For this review, take the finished solid that the model builds, in its own axes (mm). Face numbers are marked on the shaded views. A direction names the side the tool comes from. Give positions to 0.01 mm unless a question says otherwise; leave off trailing zeros. Write each loop counter-clockwise with the first axis right and the second up, starting at its lowest first coordinate (ties: lowest second). Pieces come first, ordered by that corner, then holes. Notation, with made-up numbers: (-30, 10) -> (26, 10) arc R8 cw to (26, 15) -> close; hole circle Ø10 at (-26.75, -16). An arc over 180 degrees is marked (long way). Return JSON: item names as keys, results as strings.
Autodesk Inventor part; units mm, degrees
ref_plane "Work Plane1" through (1.525, 0, 0) normal (0, 0, 1) x (1, 0, 0)
ref_plane "YZ Plane" through (0, 0, 0) normal (1, 0, 0) x (0, 1, 0)
ref_plane "XZ Plane" through (0, 0, 0) normal (0, 1, 0) x (-1, 0, 0)
sketch "Sketch1" plane through (0, 0, 0) normal (0, 0, 1) x (1, 0, 0)
  line L0 (0, 15) -> (0, 10)
  line L1 (7.5, 10) -> (80, 10)
  line L2 (80, 10) -> (80, 0)
  line L3 (80, 0) -> (-0.8001, 0)
  line L4 (-16.9601, 0) -> (96.16, 0)
  line L5 (-0.8001, 0) -> (-0.8001, 15)
  line L6 (-0.8001, 15) -> (0, 15)
  line L7 (7.5, 10) -> (5.9663, 10)
  line L8 (5.9663, 10) -> (0, 10)
  line L9 (0, -3) -> (0, 18)
  dimension "d0" = 80
  dimension "d1" = 72.5
  dimension "d2" = 20
  dimension "d9" = 0.8001
  dimension "d10" = 30
  dimension "d13" = 1.5337
  dimension "d14" = 20
revolve "Body" add sketch "Sketch1" angle 360 about axis through (80, 0, 0) along (-1, 0, 0)
sketch "Sketch2" plane through (-0.8001, 0, 0) normal (-1, 0, 0) x (0, 0, 1)
  line L0 (0, 17.3205) -> (15, 8.6603)
  line L1 (15, 8.6603) -> (15, -8.6603)
  line L2 (15, -8.6603) -> (0, -17.3205)
  line L3 (0, -17.3205) -> (-15, -8.6603)
  line L4 (-15, -8.6603) -> (-15, 8.6603)
  line L5 (-15, 8.6603) -> (0, 17.3205)
  point P0 (0, 0)
  point P1 (0, 0)
  dimension "d11" = 30
extrude "Head" add sketch "Sketch2" along normal blind 11.7
sketch "Sketch4" plane through (0, 0, 0) normal (0, 0, 1) x (1, 0, 0)
  line L0 (-12.5001, 15) -> (-12.5001, 17.3205)
  line L1 (-12.5001, 17.3205) -> (-11.1604, 17.3205)
  line L2 (-11.1604, 17.3205) -> (-12.5001, 15)
  line L3 (-14.8401, 0) -> (1.5399, 0)
  line L4 (-0.8001, 17.3205) -> (-12.5001, 17.3205)
  line L5 (-12.5001, 8.6603) -> (-12.5001, 17.3205)
  dimension "d5" = 30
  dimension "d19" = 30
revolve "Chamfer1" cut sketch "Sketch4" angle 360 about axis through (-10, 0, 0) along (1, 0, 0)
thread "Thread"
chamfer "Chamfer2" distance 1.5336 distance2 1.5337 1 edges at (80, -10, 0) measured on face at (80, -2.8768, 3.7595)
ref_plane "Work Plane1" through (1.525, 0, 0) normal (0, 0, 1) x (1, 0, 0)
sketch "Sketch7" plane through (-12.5001, 0, 0) normal (-1, 0, 0) x (0, 0, 1)
  circle A0 centre (0, 0) radius 4.5
  dimension "d59" = 9
extrude "Extrusion5" cut sketch "Sketch7" against normal blind 45
equation "\"d11\" = SW"
equation "\"d3\" = KOH - SD"
equation "\"d15\" = GEL"
equation "\"d6\" = -0.5 * SPD + 0.5 * GD"
equation "\"d0\" = NLG"
equation "\"d1\" = GEL"
equation "\"d2\" = GD"
equation "\"d10\" = SD2"
equation "\"d14\" = BDM"
equation "\"d5\" = ANG1"
equation "\"d19\" = SW0"
equation "\"NLG\" = 80"
equation "\"GD\" = NND"
equation "\"BDM\" = NND"
equation "\"KOH\" = 12.5"
equation "\"GEL\" = 72.5"
equation "\"SW\" = 30"
equation "\"SW0\" = SW"
equation "\"SPD\" = NND - 1.2269 * PTC"
equation "\"SD2\" = SW"
equation "\"SD\" = 0.8"
equation "\"ANG1\" = 30deg"
equation "\"GAL\" = 0.61345 * PTC"
equation "\"GUL\" = 0.61345 * PTC"
equation "\"RR\" = 0.8"
equation "\"WFT\" = SD"
equation "\"GD1\" = THREADDIA - 1.2269 * PTC"
equation "\"TOA\" = 30deg"
equation "\"FAWI\" = 45deg"
equation "\"PTC\" = 2.5"
equation "\"E0\" = 1.155 * SW"
properties part number "AS 1110 - M20 x 80" material "Steel, Mild"
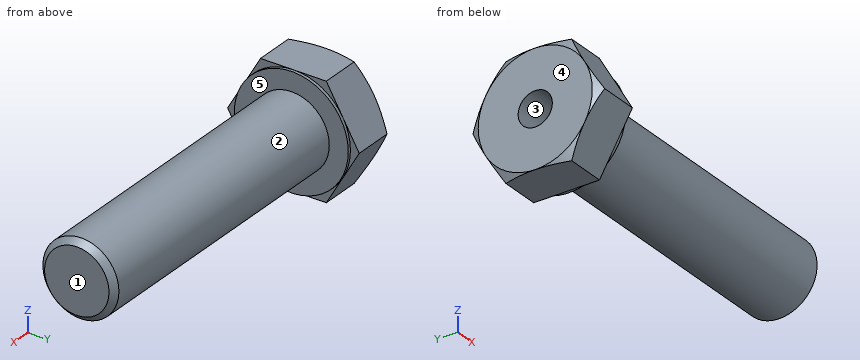
1. To check wall thickness, follow probe 1 along Y at (x, z) = (11, 0); probe 2 along X at (y, z) = (1.5, 12); probe 3 along X at (y, z) = (3, -2.5). State the ranges of each line that lie inside material, in increasing order.
Results found:
{"probe 1": "y = -10 to -4.5, 4.5 to 10", "probe 2": "x = -12.5 to 0", "probe 3": "x = 32.5 to 80"}
2. Add section A-A, the plane x = -2. State the section outline as (y, z) points, plus the area to 3 significant figures.
Results found:
{"outline": "(-17.32, 0) -> (-8.66, -15) -> (8.66, -15) -> (17.32, 0) -> (8.66, 15) -> (-8.66, 15) -> close; hole circle Ø9 at (0, 0)", "area": "716 mm²"}
3. The part is to be moulded in two halves that separate along Z. For the marked faces 1, 2 and 3, say which applies: +Z half, -Z half, draft (parallel to the pull), parting line (faces both ways), or undercut.
Results found:
{"face 1": "draft", "face 2": "parting line", "face 3": "undercut"}
4. For the marked faces 4 and 5, list the 3-axis set-ups (+Z, -Z, +X, -X, +Y, -Y) from which the entire face can be reached by the end or side of a thin tool; tool diameter is ignored.
Results found:
{"face 4": "+Z, -Z, -X, +Y, -Y", "face 5": "+X"}
5. Add section C-C, the plane x = 12. State the section outline as (y, z) points, plus the area to 3 significant figures.
Results found:
{"outline": "circle Ø20 at (0, 0); hole circle Ø9 at (0, 0)", "area": "251 mm²"}
6. Add section B-B, the plane x = 68.5. State the section outline as (y, z) points, plus the area to 3 significant figures.
Results found:
{"outline": "circle Ø20 at (0, 0)", "area": "314 mm²"}
7. For pin 1 (4 mm diameter, centred on y = 13.5, z = -9, fed in from +X); pin 2 (5 mm diameter, centred on x = 4.5, y = 2, fed in from -Z); pin 3 (6 mm diameter, centred on y = -3.5, z = 12, fed in from +X), all flat-tipped, find the tip position at first contact; note any pin that passes through.
Results found:
{"pin 1": "stops at x = 0", "pin 2": "stops at z = -10", "pin 3": "stops at x = 78.97"}
